Read the model definition and answer for the solid it produces. Units are mm, in the model's axes. A direction names the side the tool comes from. Give positions to 0.01 mm unless a question says otherwise; leave off trailing zeros. Order: outer loops, then holes, each group sorted by start corner. A loop starts at its lowest first (then second) coordinate and runs counter-clockwise, first axis right, second up. Notation, with made-up numbers: (14, 63.25) - (49, 63.25) arc R6 cw to (49, 67.25) - close; hole circle Ø5 at (89, 14.5). An arc over 180 degrees is marked (long way). Use a Markdown table: item, result. Add a question column.
1. For a pull along X with two mould halves and no side action, classify faces 4 (the cylindrical face through (-11.19, 1.23, 0.49)), 5 (the flat face through (21.5, -9, 23)), 6 (the flat face through (0, -37, 41)), 7 (the cylindrical face through (18.032, 1.232, -16.843)) as released by +X, released by -X, zero draft, split by the parting line, or undercut.
2. A cutting plane is placed at A-A on x = 0. Determine the outline of the cut face in (y, z), and give its area (3 significant figures).
3. Consider L1, parallel to X at y = 1.9, z = 16; L2, parallel to Y at x = 0, z = -18; L3, parallel to X at y = 12.5, z = -20.4. Determine where each line is inside the solid, lowest interval first.
4. A cutting plane is placed at C-C on z = 16. Determine the outline of the cut face in (x, y), and give its area (3 significant figures).
5. A cutting plane is placed at B-B on y = 1.5. Determine the outline of the cut face in (x, z), and give its area (3 significant figures).
6. Which of the six approach directions +Z, -Z, +X, -X, +Y, -Y give full straight-line access (tool end or side, diameter ignored) to faces 1 (the flat face through (9, 0, 9)), 2 (the flat face through (0, 9, -16.5)), 3 (the flat face through (-8, -38, 33))?
7. Flat-ended cylindrical pins translate along their axes: P1, Ø16.5, axis at x = -1, z = 35.5, coming from the +Y side; P2, Ø1.5, axis at x = -1.5, y = -29.5, coming from the -Z side; P3, Ø10, axis at x = 10, y = -15.5, coming from the +Z side; P4, Ø6.5, axis at x = 0, z = 33, coming from the -Y side. Find the tip coordinate at first contact, or state that the pin passes through.
8. A cutting plane is placed at D-D on x = -16. Determine the outline of the cut face in (y, z).
Autodesk Fusion 360 part; units mm, degrees
sketch "Sketch1" plane through (0, 0, 0) normal (0, 1, 0) x (1, 0, 0)
  circle A0 centre (0, 0) radius 11.2
  line L0 (21.5, 21.5) -> (-21.5, 21.5)
  line L1 (-21.5, 21.5) -> (-21.5, -21.5)
  line L2 (-21.5, -21.5) -> (21.5, -21.5)
  line L3 (21.5, -21.5) -> (21.5, 21.5)
  line L4 (21.5, 21.5) -> (-21.5, -21.5) construction
  line L5 (-21.5, 21.5) -> (21.5, -21.5) construction
  line L6 (21.5, 21.5) -> (16, 21.5)
  line L7 (16, 21.5) -> (16, 16)
  circle A1 centre (16, 16) radius 2.2
  circle A2 centre (-16, 16) radius 2.2
  circle A3 centre (-16, -16) radius 2.2
  circle A4 centre (16, -16) radius 2.2
  line L8 (26, 26) -> (-26, 26)
  line L9 (-26, 26) -> (-26, -26)
  line L10 (-26, -26) -> (26, -26)
  line L11 (26, -26) -> (26, 26)
  line L12 (26, 26) -> (-26, -26) construction
  line L13 (-26, 26) -> (26, -26) construction
  line L14 (-21.5, -21.5) -> (-26, -21.5)
  line L15 (21.5, -21.5) -> (26, -21.5)
  line L16 (-21.5, 21.5) -> (-26, 21.5)
  line L17 (21.5, 21.5) -> (26, 21.5)
  dimension "d1" = 22.4
  dimension "d2" = 43
  dimension "d3" = 43
  dimension "d4" = 5.5
  dimension "d5" = 5.5
  dimension "d6" = 4.4
  dimension "d8" = 360
  dimension "d9" = 52
  dimension "d10" = 52
extrude "Extrude1" add sketch "Sketch1" along normal blind 5
extrude "Extrude7" add sketch "Sketch1" against normal blind 40 contours L2 L9 L10 L11 L14 L15
extrude "Extrude8" cut sketch "Sketch1" along normal blind 32 contours L0 L6 L8 L9 L11 L16 L17
sketch "Sketch7" plane through (0, 5, 0) normal (0, 1, 0) x (-1, 0, 0)
  line L0 (-26, -21.5) -> (26, -21.5)
  line L1 (26, -21.5) -> (26, 26)
  line L2 (26, 26) -> (-26, 26)
  line L3 (-26, 26) -> (-26, -21.5)
  circle A0 centre (16, 16) radius 2.2
  circle A1 centre (-16, 16) radius 2.2
  circle A2 centre (16, -16) radius 2.2
  circle A3 centre (0, 0) radius 11.2
  circle A4 centre (-16, -16) radius 2.2
  line L4 (0, -21.5) -> (8, -21.5)
  line L5 (8, -21.5) -> (-8, -21.5)
  line L6 (-8, -21.5) -> (-8, -16.5)
  line L7 (-8, -16.5) -> (8, -16.5)
  line L8 (8, -16.5) -> (8, -21.5)
  dimension "d48" = 8
  dimension "d49" = 16
  dimension "d50" = 5
extrude "Extrude9" add sketch "Sketch7" along normal blind 15 contours L0 L4 L5 L6 L7 L8
sketch "Sketch8" plane through (0, 0, -16.5) normal (0, 0, 1) x (1, 0, 0)
  line L0 (-8, 5) -> (8, 5)
  line L1 (8, 5) -> (8, 20)
  line L2 (8, 20) -> (-8, 20)
  line L3 (-8, 20) -> (-8, 5)
  line L4 (0, 20) -> (0, 12.5)
  circle A0 centre (0, 12.5) radius 2.75
  dimension "d53" = 5.5
extrude "Extrude10" cut sketch "Sketch8" against normal blind 14 contours A0
sketch "Sketch9" plane through (0, 0, 26) normal (0, 0, 1) x (1, 0, 0)
  line L0 (26, -40) -> (26, 5)
  line L1 (26, 5) -> (-26, 5)
  line L2 (-26, 5) -> (-26, -40)
  line L3 (-26, -40) -> (26, -40)
  line L4 (0, -40) -> (8, -40)
  line L5 (8, -40) -> (-8, -40)
  line L6 (-8, -40) -> (-8, -35)
  line L7 (-8, -35) -> (8, -35)
  line L8 (8, -35) -> (8, -40)
  dimension "d56" = 8
  dimension "d57" = 16
  dimension "d58" = 5
extrude "Extrude11" add sketch "Sketch9" along normal blind 15 contours L3 L4 L5 L6 L7 L8
sketch "Sketch10" plane through (0, -35, 0) normal (0, 1, 0) x (-1, 0, 0)
  line L0 (-8, 26) -> (8, 26)
  line L1 (8, 26) -> (8, 41)
  line L2 (8, 41) -> (-8, 41)
  line L3 (-8, 41) -> (-8, 26)
  line L4 (0, 41) -> (0, 33)
  circle A0 centre (0, 33) radius 2.75
  dimension "d61" = 5.5
extrude "Extrude12" cut sketch "Sketch10" against normal blind 11 contours A0
extrude "Extrude13" cut sketch "Sketch1" along normal blind 6 contours L3 L11 L15 L17 | L1 L9 L14 L16
sketch "Sketch11" plane through (0, 0, 21.5) normal (0, 0, -1) x (-1, 0, 0)
  line L0 (-26, 5) -> (-26, -40)
  line L1 (-26, -40) -> (26, -40)
  line L2 (26, -40) -> (26, 5)
  line L3 (26, 5) -> (21.5, 5)
  line L4 (21.5, 5) -> (21.5, 0)
  line L5 (21.5, 0) -> (-21.5, 0)
  line L6 (-21.5, 0) -> (-21.5, 5)
  line L7 (-21.5, 5) -> (-26, 5)
  line L8 (21.5, 0) -> (21.5, -40)
  line L9 (-21.5, 0) -> (-21.5, -40)
extrude "Extrude14" cut sketch "Sketch11" against normal blind 15 contours L0 L1 L6 L7 L9 | L1 L2 L3 L4 L8
extrude "Extrude15" cut 1 faces at (4.8761, 5, 23.24) along direction (0, -1, 0) blind 2.5
Output values:
| question | item | result |
|---|---|---|
| 1 | face 4 | undercut |
| 1 | face 5 | released by +X |
| 1 | face 6 | zero draft |
| 1 | face 7 | undercut |
| 2 | outline | (-40, 21.5) - (0, 21.5) - (0, 11.2) - (2.5, 11.2) - (2.5, 26) - (-35, 26) - (-35, 30.25) - (-40, 30.25) - close; (-40, 35.75) - (-35, 35.75) - (-35, 41) - (-40, 41) - close; (0, -21.5) - (9.75, -21.5) - (9.75, -16.5) - (2.5, -16.5) - (2.5, -11.2) - (0, -11.2) - close; (15.25, -21.5) - (20, -21.5) - (20, -16.5) - (15.25, -16.5) - close |
| 2 | area | 350 mm² |
| 3 | L1 | -21.5 to -18.2, -13.8 to 13.8, 18.2 to 21.5 |
| 3 | L2 | 0 to 9.75, 15.25 to 20 |
| 3 | L3 | -8 to -2.75, 2.75 to 8 |
| 4 | outline | (-21.5, 0) - (-18.2, 0) - (-18.2, 2.5) - (-21.5, 2.5) - close; (-13.8, 0) - (13.8, 0) - (13.8, 2.5) - (-13.8, 2.5) - close; (18.2, 0) - (21.5, 0) - (21.5, 2.5) - (18.2, 2.5) - close |
| 4 | area | 85.5 mm² |
| 5 | outline | (-21.5, -21.5) - (21.5, -21.5) - (21.5, 26) - (-21.5, 26) - close; hole circle Ø4.4 at (-16, -16); hole circle Ø4.4 at (-16, 16); hole circle Ø22.4 at (0, 0); hole circle Ø4.4 at (16, -16); hole circle Ø4.4 at (16, 16) |
| 5 | area | 1,590 mm² |
| 6 | face 1 | -Z, +X, -X, -Y |
| 6 | face 2 | +Z, +X, -X, +Y |
| 6 | face 3 | +Z, -X, +Y, -Y |
| 7 | P1 | y = -35 |
| 7 | P2 | z = 21.5 |
| 7 | P3 | z = 26 |
| 7 | P4 | y = -40 |
| 8 | outline | (-40, 21.5) - (0, 21.5) - (0, 18.2) - (2.5, 18.2) - (2.5, 26) - (-40, 26) - close; (0, -21.5) - (2.5, -21.5) - (2.5, -18.2) - (0, -18.2) - close; (0, -13.8) - (2.5, -13.8) - (2.5, 13.8) - (0, 13.8) - close |
